The listing builds one solid part. Answer for the finished solid, in the listing's coordinates (mm). Face numbers are marked on the shaded views. A direction names the side the tool comes from. Coordinates: 2 decimals unless noted, no trailing zeros. Loops run counter-clockwise (first coordinate to the right, second up) from the corner with the lowest first, then second, coordinate; pieces in that order, holes last. Notation, with made-up numbers: M 56,58.25 L 91,58.25 A25 cw 91,83.25 Z; hole C -30.75,87.25 d2. An arc over 180 degrees is marked long. Answer as CSV lines item,"result". Start each with the question number.
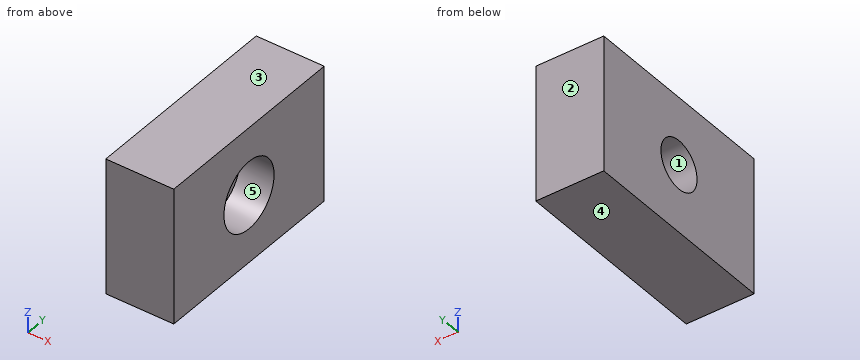
```python
from build123d import *

# Parameters (mm, degrees)
F0_W     = 150
F0_H     = 100
F0_R     = 25
F0_R_2   = 18
F1_DEPTH = 25
F2_DEPTH = 50


with BuildPart() as f1:
    # F0 (on Right) → F1 (new body)
    with BuildSketch(Plane.YZ):
        Rectangle(F0_W, F0_H)
        Circle(F0_R, mode=Mode.SUBTRACT)
        Circle(F0_R)
        Circle(F0_R_2, mode=Mode.SUBTRACT)
    extrude(amount=F1_DEPTH)

    # F0 (on Right) → F2 (join)
    with BuildSketch(Plane.YZ):
        Rectangle(F0_W, F0_H)
        Circle(F0_R, mode=Mode.SUBTRACT)
    extrude(amount=F2_DEPTH)


solid = f1.part
```
Item 1: Consider line 1 (Y direction, x = 34.75, z = 0); line 2 (Z direction, x = 34.5, y = 0); line 3 (Y direction, x = 11.5, z = -9). Determine where each line is inside the solid, lowest interval first.
Item 2: Each of these flat-tipped pins is pushed along its axis until it touches: P1, Ø25, axis at y = 8.5, z = 7, coming from the +X side; P2, Ø1.5, axis at y = -28, z = 22, coming from the -X side. Where does it stop, or does it pass through?
Item 3: Section C-C on y = 0 is taken. Determine the outline of the cut face in (x, z), then the cut area to 3 significant figures.
Item 4: Section D-D on x = 35 is taken. Determine the outline of the cut face in (y, z).
Item 5: For a pull along Z with two mould halves and no side action, classify the marked faces 1, 2 and 3 as pulls with the +Z half, pulls with the -Z half, needs draft (parallel to the pull), parting line crosses it, or undercut.
Item 6: Section B-B on x = 20 is taken. Determine the outline of the cut face in (y, z), then the cut area to 3 significant figures.
Item 7: Section A-A on z = 0 is taken. Determine the outline of the cut face in (x, y), then the cut area to 3 significant figures.
Item 8: For the marked faces 4 and 5, determine the directions among +Z, -Z, +X, -X, +Y, -Y from which every point of the face is accessible in a straight line to the end or side of a thin tool.
Results are:
1,line 1,"-75 to -25, 25 to 75"
1,line 2,"-50 to -25, 25 to 50"
1,line 3,"-75 to -15.59, 15.59 to 75"
2,P1,"x = 25"
2,P2,"x = 0"
3,outline,"M 0,-50 L 50,-50 L 50,-25 L 25,-25 L 25,-18 L 0,-18 Z; M 0,18 L 25,18 L 25,25 L 50,25 L 50,50 L 0,50 Z"
3,area,"2,850 mm²"
4,outline,"M -75,-50 L 75,-50 L 75,50 L -75,50 Z; hole C 0,0 d50"
5,face 1,"undercut"
5,face 2,"needs draft"
5,face 3,"pulls with the +Z half"
6,outline,"M -75,-50 L 75,-50 L 75,50 L -75,50 Z; hole C 0,0 d36"
6,area,"14,000 mm²"
7,outline,"M 0,-75 L 50,-75 L 50,-25 L 25,-25 L 25,-18 L 0,-18 Z; M 0,18 L 25,18 L 25,25 L 50,25 L 50,75 L 0,75 Z"
7,area,"5,350 mm²"
8,face 4,"-Z, +X, -X, +Y, -Y"
8,face 5,"+X"
